```python
from build123d import *

# Parameters (mm, degrees)
F1_DEPTH = 23
F2_T     = -1.9
F4_DEPTH = 2
F5_R     = 1.4
F6_DEPTH = 2
F7_R     = 1.4
F8_DEPTH = 2


with BuildPart() as f1:
    # F0 (on Top) → F1 (new body)
    with BuildSketch(Plane.XY):
        with BuildLine():
            Line((-36, -67), (36, -67))
            ThreePointArc((36, -67), (39.535534, -65.535534), (41, -62))
            Line((41, -62), (41, 62))
            ThreePointArc((41, 62), (39.535534, 65.535534), (36, 67))
            Line((36, 67), (-36, 67))
            ThreePointArc((-36, 67), (-39.535534, 65.535534), (-41, 62))
            Line((-41, 62), (-41, -62))
            ThreePointArc((-41, -62), (-39.535534, -65.535534), (-36, -67))
        make_face()
    extrude(amount=F1_DEPTH)

    # F2
    f2_openings = [f1.faces().sort_by_distance(p)[0] for p in [
        (0, 0, 23),
    ]]
    offset(amount=F2_T, openings=f2_openings)

    # F3 (on face) → F4 (cut)
    with BuildSketch(Plane.XY.offset(1.9)):
        with BuildLine():
            ThreePointArc((15.5, 3.5), (18, 1), (20.5, 3.5))
            Line((20.5, 3.5), (20.5, 10.5))
            ThreePointArc((20.5, 10.5), (18, 13), (15.5, 10.5))
            Line((15.5, 10.5), (15.5, 3.5))
        make_face()
    extrude(amount=-F4_DEPTH, mode=Mode.SUBTRACT)

    # F5 (on face) → F6 (cut)
    with BuildSketch(Plane(origin=(-41, 0, 0), x_dir=(0, -1, 0), z_dir=(-1, 0, 0))):
        with Locations((-45, 17)):
            Circle(F5_R)
        with Locations((45, 17)):
            Circle(F5_R)
    extrude(amount=-F6_DEPTH, mode=Mode.SUBTRACT)

    # F7 (on face) → F8 (cut)
    with BuildSketch(Plane.YZ.offset(41)):
        with Locations((-55, 17)):
            Circle(F7_R)
        with Locations((45, 17)):
            Circle(F7_R)
    extrude(amount=-F8_DEPTH, mode=Mode.SUBTRACT)


solid = f1.part
```
Here's how the part is built. I have some questions about the finished solid (model axes, mm). A direction names the side the tool comes from. Round coordinates to 2 decimals unless told otherwise and drop trailing zeros. Order: outer loops, then holes, each group sorted by start corner. A loop starts at its lowest first (then second) coordinate and runs counter-clockwise, first axis right, second up. Notation, with made-up numbers: M -34.5,76 L 2.5,76 A27 ccw 2.5,110 Z; hole C 87.25,24 d11. An arc over 180 degrees is marked long. Answer as CSV lines item,"result".
Item 1: Which directions (+Z, -Z, +X, -X, +Y, -Y) give clear straight access to the entire face, cutting with the end or side of a thin tool? Please do faces 4 (the cylindrical face through (38.216, 64.168, 12.302)), 5 (the flat face through (1, 67, 11)), 6 (the cylindrical face through (18, 1, 1)).
From the geometry:
face 4,"+Z"
face 5,"+Z, -Z, +X, -X, +Y"
face 6,"+Z, -Z"
Item 2: Please list where these lines run through material, in increasing order: L1, parallel to X at y = -16.5, z = 5.5; L2, parallel to Z at x = 40.65, y = -55; L3, parallel to Y at x = 19.5, z = 3.75. Write a range as [from, to].
From the geometry:
L1,"[-41, -39.1], [39.1, 41]"
L2,"[0, 15.6], [18.4, 23]"
L3,"[-67, -65.1], [65.1, 67]"
Item 3: Imagine slicing it at A-A on z = 17. Give the number of separate pieces and of enclosed holes in the cut face, and give its area (3 significant figures).
From the geometry:
separate pieces,"4"
enclosed holes,"0"
area,"772 mm2"
Item 4: Imagine slicing it at D-D on y = 45. List the corners of the cut face in (x, z) for me, and give its area (3 significant figures).
From the geometry:
outline,"M -41,0 L 41,0 L 41,15.6 L 39.1,15.6 L 39.1,1.9 L -39.1,1.9 L -39.1,15.6 L -41,15.6 Z; M -41,18.4 L -39.1,18.4 L -39.1,23 L -41,23 Z; M 39.1,18.4 L 41,18.4 L 41,23 L 39.1,23 Z"
area,"225 mm2"
Item 5: We'd pull the mould along Y, two halves only. Please class faces 1 (the flat face through (-1, 1, 0)), 2 (the cylindrical face through (39, -66, 11)), 3 (the cylindrical face through (18, 13, 1)): +Y half, -Y half, draft (parallel to the pull), parting line (faces both ways), or undercut.
From the geometry:
face 1,"draft"
face 2,"-Y half"
face 3,"undercut"
Item 6: For pin 1 (2.5 mm diameter, centred on y = -45, z = 17, fed in from -X); pin 2 (3 mm diameter, centred on y = 45, z = 17, fed in from -X); pin 3 (1.7 mm diameter, centred on y = 45, z = 17, fed in from -X), each with a flat end and sliding along its axis, tell me the tip position at first contact or that it passes through.
From the geometry:
pin 1,"x = 39.1"
pin 2,"x = -41"
pin 3,"through"
Item 7: Imagine slicing it at B-B on y = -45. List the corners of the cut face in (x, z) for me, and give its area (3 significant figures).
From the geometry:
outline,"M -41,0 L 41,0 L 41,23 L 39.1,23 L 39.1,1.9 L -39.1,1.9 L -39.1,15.6 L -41,15.6 Z; M -41,18.4 L -39.1,18.4 L -39.1,23 L -41,23 Z"
area,"231 mm2"
Item 8: Imagine slicing it at C-C on x = 18. List the corners of the cut face in (y, z) for me, and give its area (3 significant figures).
From the geometry:
outline,"M -67,0 L 1,0 L 1,1.9 L -65.1,1.9 L -65.1,23 L -67,23 Z; M 13,0 L 67,0 L 67,23 L 65.1,23 L 65.1,1.9 L 13,1.9 Z"
area,"312 mm2"
